Design review of the part built by this model. Coordinates are the model's own, in mm. A direction names the side the tool comes from. Give positions to 0.01 mm unless a question says otherwise; leave off trailing zeros. Loops run counter-clockwise (first coordinate to the right, second up) from the corner with the lowest first, then second, coordinate; pieces in that order, holes last. Notation, with made-up numbers: (79, 61) - (85, 61) arc R13 cw to (85, 77) - close; hole circle Ø2 at (-17, 66.5). An arc over 180 degrees is marked (long way). Write each question's results on one line, items separated by ' | '.
```python
from build123d import *

# Parameters (mm, degrees)
F0_W     = 73.0307288468
F0_H     = 76.5502825379
F1_DEPTH = 20
F2_W     = 12.9050291143
F2_H     = 25.5167605355
F3_DEPTH = 10
F5_D     = 2.794


with BuildPart() as f1:
    # F0 (on Front) → F1 (new body)
    with BuildSketch(Plane.XZ):
        with Locations((0.7332395762, -0.586591661)):
            Rectangle(F0_W, F0_H)
    extrude(amount=F1_DEPTH)

    # F2 (on face) → F3 (cut)
    with BuildSketch(Plane(origin=(0, 0, 0), x_dir=(-1, 0, 0), z_dir=(0, 1, 0))):
        with Locations((-0.2932955977, -1.4664805494)):
            Rectangle(F2_W, F2_H)
    extrude(amount=-F3_DEPTH, mode=Mode.SUBTRACT)

    # F5 (through all)
    with Locations(Plane.XZ.offset(20)):
        with Locations((0, 25.6550256172), (-25.6550256172, 0), (0, -25.6550256172), (25.6550256172, 0)):
            Hole(F5_D / 2)


solid = f1.part
```
Item 1: We need section B-B on z = 0. Give the boundary of the cut face in (x, y), then the cut area to 3 significant figures.
Output values:
outline: (-35.78, -20) - (-27.05, -20) - (-27.05, 0) - (-35.78, 0) - close; (-24.26, -20) - (24.26, -20) - (24.26, 0) - (6.75, 0) - (6.75, -10) - (-6.16, -10) - (-6.16, 0) - (-24.26, 0) - close; (27.05, -20) - (37.25, -20) - (37.25, 0) - (27.05, 0) - close | area: 1,220 mm²
Item 2: Clearance check with flat-ended pins moving along their axes: P1, Ø10, axis at x = 23, z = 5, coming from the +Y side; P2, Ø2.5, axis at x = -25.66, z = 0, coming from the +Y side (3 decimals). State where each tip first meets the part, or that it passes through.
Output values:
P1: stops at y = 0 | P2: passes through
Item 3: Draft analysis for pull direction Z (two halves, no side actions). For faces 3 (the face through (-24.546, -9.86, -0.85)), 4 (the face through (-35.782, -10, -1)), 5 (the face through (0, -10, 37.689)), state which applies: +Z half, -Z half, draft (parallel to the pull), parting line (faces both ways), or undercut.
Output values:
face 3: undercut | face 4: draft | face 5: +Z half
Item 4: We need section A-A on x = 0. Give the boundary of the cut face in (y, z), then the cut area to 3 significant figures.
Output values:
outline: (-20, -38.86) - (0, -38.86) - (0, -27.05) - (-20, -27.05) - close; (-20, -24.26) - (0, -24.26) - (0, -14.22) - (-10, -14.22) - (-10, 11.29) - (0, 11.29) - (0, 24.26) - (-20, 24.26) - close; (-20, 27.05) - (0, 27.05) - (0, 37.69) - (-20, 37.69) - close | area: 1,160 mm²
Item 5: Tool access review of faces 1 (the face through (0, -5, 11.292)), 2 (the face through (24.323, -9.86, 0.42)): name each direction out of +Z, -Z, +X, -X, +Y, -Y from which nothing blocks a thin tool from reaching the whole face with its end or side.
Output values:
face 1: +Y | face 2: +Y, -Y
Item 6: We need section D-D on y = -3. Give the boundary of the cut face in (x, z).
Output values:
outline: (-35.78, -38.86) - (37.25, -38.86) - (37.25, 37.69) - (-35.78, 37.69) - close; hole circle Ø2.79 at (-25.66, 0); hole (-6.16, -14.22) - (6.75, -14.22) - (6.75, 11.29) - (-6.16, 11.29) - close; hole circle Ø2.79 at (0, -25.66); hole circle Ø2.79 at (0, 25.66); hole circle Ø2.79 at (25.66, 0)
Item 7: We need section C-C on z = -12.5. Give the boundary of the cut face in (x, y), then the cut area to 3 significant figures.
Output values:
outline: (-35.78, -20) - (37.25, -20) - (37.25, 0) - (6.75, 0) - (6.75, -10) - (-6.16, -10) - (-6.16, 0) - (-35.78, 0) - close | area: 1,330 mm²
Item 8: Wall thickness on probe 1 along Z at (x, y) = (0, -7.5); probe 2 along X at (y, z) = (-4, -1.5); probe 3 along X at (y, z) = (-3.75, 26.5): over which ranges is each line inside the solid? List them lowest first.
Output values:
probe 1: z = -38.86 to -27.05, -24.26 to -14.22, 11.29 to 24.26, 27.05 to 37.69 | probe 2: x = -35.78 to -6.16, 6.75 to 37.25 | probe 3: x = -35.78 to -1.11, 1.11 to 37.25
